Check sheet for the modelled part. Datum: model origin and axes. Units: mm. A direction names the side the tool comes from. Give positions to 0.01 mm unless a question says otherwise; leave off trailing zeros. Write each loop counter-clockwise with the first axis right and the second up, starting at its lowest first coordinate (ties: lowest second). Pieces come first, ordered by that corner, then holes. Notation, with made-up numbers: M 70,22.5 L 124,22.5 A30 cw 124,50.5 Z; hole C -29,51 d5. An arc over 180 degrees is marked long. Write item = value, one per line. Start each with the question number.
1) Scan lines: line 1 along X through (y, z) = (4.1, 0); line 2 along Y through (x, z) = (2, 0.5); line 3 along X through (y, z) = (5.1, -5.25). Record each from-to range of solid material in increasing order. Write a range as [from, to].
2) Cross-section at C-C, the plane y = 2.05. Record the cut outline in (x, z), plus the area to 3 significant figures.
3) Go/stop test with a flat-tipped pin: pin 1 (1.5 mm diameter, centred on y = 2, z = -3, fed in from -X). Record where the tip stops, or that it passes through.
4) Cross-section at B-B, the plane z = 0. Record the cut outline in (x, y).
5) Access from +Z, -Z, +X, -X, +Y, -Y to the whole of each face (thin tool, end or side, straight path). Record for faces 4 (the flat face through (7, 6, -1)), 5 (the cylindrical face through (2.058, 3.465, 6.534)).
6) Cross-section at A-A, the plane x = 0. Record the cut outline in (y, z).
7) Mould release check, pull along Z, two halves, no side actions. Record for faces 1 (the cylindrical face through (0.44, 0.49, -10.04)), 2 (the flat face through (0, 0, 0)), 3 (the flat face through (0, 1, 0)): released by +Z, released by -Z, zero draft, split by the parting line, or undercut.
```python
from build123d import *

# Parameters (mm, degrees)
SKETCH1_R           = 10.05
BOSS_EXTRUDE1_DEPTH = 1
SKETCH2_R           = 8.85
SKETCH2_R_2         = 6.85
BOSS_EXTRUDE2_DEPTH = 5
BOSS_EXTRUDE4_START = -5
SKETCH3_R           = 8.95
SKETCH3_R_2         = 6.85
BOSS_EXTRUDE4_DEPTH = 5
BOSS_EXTRUDE5_START = -5
SKETCH4_R           = 9.01
SKETCH4_R_2         = 6.85
BOSS_EXTRUDE5_DEPTH = 5


with BuildPart() as part:
    # Sketch1 → Boss-Extrude1 (new body)
    with BuildSketch(Plane(origin=(0, 0, 0), x_dir=(1, 0, 0), z_dir=(0, 1, 0))):
        with Locations(Location((0, 0, 0), (0, 0, 270))):
            Circle(SKETCH1_R)
    extrude(amount=BOSS_EXTRUDE1_DEPTH)

    # Sketch2 → Boss-Extrude2 (add)
    with BuildSketch(Plane(origin=(0, 1, 0), x_dir=(1, 0, 0), z_dir=(0, 1, 0))):
        with Locations(Location((0, 0, 0), (0, 0, 270))):
            Circle(SKETCH2_R)
        with Locations(Location((0, 0, 0), (0, 0, 270))):
            Circle(SKETCH2_R_2, mode=Mode.SUBTRACT)
    extrude(amount=BOSS_EXTRUDE2_DEPTH)

    # Sketch3 → Boss-Extrude4 (add)
    with BuildSketch(Plane(origin=(0, 6, 0), x_dir=(1, 0, 0), z_dir=(0, 1, 0)).offset(BOSS_EXTRUDE4_START)):
        with Locations(Location((0, 0, 0), (0, 0, 270))):
            Circle(SKETCH3_R)
        with Locations(Location((0, 0, 0), (0, 0, 270))):
            Circle(SKETCH3_R_2, mode=Mode.SUBTRACT)
    extrude(amount=BOSS_EXTRUDE4_DEPTH)

    # Sketch4 → Boss-Extrude5 (add)
    with BuildSketch(Plane(origin=(0, 6, 0), x_dir=(1, 0, 0), z_dir=(0, 1, 0)).offset(BOSS_EXTRUDE5_START)):
        with Locations(Location((0, 0, 0), (0, 0, 270))):
            Circle(SKETCH4_R)
        with Locations(Location((0, 0, 0), (0, 0, 270))):
            Circle(SKETCH4_R_2, mode=Mode.SUBTRACT)
    extrude(amount=BOSS_EXTRUDE5_DEPTH)


solid = part.part
```
Reply:
q1.line_1 = [-9.01, -6.85], [6.85, 9.01]
q1.line_2 = [0, 1]
q1.line_3 = [-7.32, -4.4], [4.4, 7.32]
q2.outline = C 0,0 d18.02; hole C 0,0 d13.7
q2.area = 108 mm2
q3.pin_1 = -8.72
q4.outline = M -10.05,0 L 10.05,0 L 10.05,1 L 9.01,1 L 9.01,6 L 6.85,6 L 6.85,1 L -6.85,1 L -6.85,6 L -9.01,6 L -9.01,1 L -10.05,1 Z
q5.face_4 = +Z, -Z, +X, -X, +Y
q5.face_5 = +Y
q6.outline = M 0,-10.05 L 1,-10.05 L 1,-9.01 L 6,-9.01 L 6,-6.85 L 1,-6.85 L 1,6.85 L 6,6.85 L 6,9.01 L 1,9.01 L 1,10.05 L 0,10.05 Z
q7.face_1 = split by the parting line
q7.face_2 = zero draft
q7.face_3 = undercut
